from build123d import *

# Parameters (mm, degrees)
BOSS_EXTRUDE1_DEPTH   = 7.2
SKETCH1_3_R           = 3.75
SKETCH1_3_R_2         = 1.6
BOSS_EXTRUDE2_DEPTH   = 2
BOSS_EXTRUDE2_2_DEPTH = 2
BOSS_EXTRUDE3_DEPTH   = 2
BOSS_EXTRUDE4_DEPTH   = 7.5
SKETCH3_R             = 3.75
CUT_EXTRUDE6_DEPTH    = 12
BOSS_EXTRUDE5_DEPTH   = 7.5
SKETCH5_R             = 3.75
CUT_EXTRUDE7_DEPTH    = 7.5
SKETCH6_W             = 29.5
SKETCH6_H             = 8.4
BOSS_EXTRUDE6_DEPTH   = 4.3
SKETCH7_W             = 7.5
SKETCH7_H             = 7.2
SKETCH7_W_2           = 16.3
BOSS_EXTRUDE7_DEPTH   = 2
SKETCH8_W             = 10.1
SKETCH8_H             = 2.3
CUT_EXTRUDE8_DEPTH    = 12
SKETCH9_W             = 10.1
SKETCH9_H             = 1.2
BOSS_EXTRUDE8_DEPTH   = 6.4
SKETCH11_W            = 9.1347476
SKETCH11_H            = 5.173710516
BOSS_EXTRUDE11_DEPTH  = 5.5
SKETCH12_R            = 3.106234899
CUT_EXTRUDE10_DEPTH   = 1.5
CUT_EXTRUDE10_DRAFT   = -25
SKETCH13_R            = 3.196774454
CUT_EXTRUDE11_DEPTH   = 1.5
CUT_EXTRUDE11_DRAFT   = -29
SKETCH14_W            = 8.1347476
SKETCH14_H            = 4.5
CUT_EXTRUDE12_DEPTH   = 4.5
SCALE1_SCALE          = 0.2


# Read off the part's stored shape, not the designer's step: Dome1, Dome2
with BuildPart() as part:
    # Sketch1 → Boss-Extrude1 (new body)
    with BuildSketch(Plane(origin=(0, 0, 0), x_dir=(1, 0, 0), z_dir=(0, 1, 0))):
        Polygon((14.75, 0), (-14.75, 0), (-14.75, -3.75), (-14.75, -6.5), (14.75, -6.5), (14.75, -3.75), align=None)
        Polygon((-14.75, 3.75), (-14.75, 0), (14.75, 0), (14.75, 3.75), (14.75, 6.5), (-14.75, 6.5), align=None)
    extrude(amount=BOSS_EXTRUDE1_DEPTH)



with BuildPart() as body_2:
    # Sketch1<3> → Boss-Extrude2 (new body)
    with BuildSketch(Plane(origin=(0, 0, 0), x_dir=(1, 0, 0), z_dir=(0, 1, 0))):
        with Locations(Location((-18.5, 0, 0), (0, 0, 270))):
            Circle(SKETCH1_3_R)
        with Locations(Location((-18.5, 0, 0), (0, 0, 270))):
            Circle(SKETCH1_3_R_2, mode=Mode.SUBTRACT)
    extrude(amount=BOSS_EXTRUDE2_DEPTH)


with BuildPart() as body_3:
    # Sketch1<3> → Boss-Extrude2 2 (new body)
    with BuildSketch(Plane(origin=(0, 0, 0), x_dir=(1, 0, 0), z_dir=(0, 1, 0))):
        with Locations(Location((18.5, 0, 0), (0, 0, 270))):
            Circle(SKETCH1_3_R)
        with Locations(Location((18.5, 0, 0), (0, 0, 270))):
            Circle(SKETCH1_3_R_2, mode=Mode.SUBTRACT)
    extrude(amount=BOSS_EXTRUDE2_2_DEPTH)


with BuildPart() as part_1:
    add(part.part)

    add(body_2.part)  # Boss-Extrude3 merges body 2

    add(body_3.part)  # Boss-Extrude3 merges body 3
    # Sketch1<4> → Boss-Extrude3 (add)
    with BuildSketch(Plane(origin=(0, 0, 0), x_dir=(1, 0, 0), z_dir=(0, 1, 0))):
        with BuildLine():
            Line((-14.75, -3.75), (-14.75, 0))
            ThreePointArc((-14.75, 0), (-15.848349571, -2.651650429), (-18.5, -3.75))
            Line((-18.5, -3.75), (-14.75, -3.75))
        make_face()
        with BuildLine():
            Line((-14.75, 0), (-14.75, 3.75))
            Line((-14.75, 3.75), (-18.5, 3.75))
            ThreePointArc((-18.5, 3.75), (-15.848349571, 2.651650429), (-14.75, 0))
        make_face()
        with BuildLine():
            Line((18.5, 3.75), (14.75, 3.75))
            Line((14.75, 3.75), (14.75, 0))
            ThreePointArc((14.75, 0), (15.848349571, 2.651650429), (18.5, 3.75))
        make_face()
        with BuildLine():
            ThreePointArc((18.5, -3.75), (15.848349571, -2.651650429), (14.75, 0))
            Line((14.75, 0), (14.75, -3.75))
            Line((14.75, -3.75), (18.5, -3.75))
        make_face()
    extrude(amount=BOSS_EXTRUDE3_DEPTH)

    # Sketch2 → Boss-Extrude4 (add)
    with BuildSketch(Plane.XY.offset(3.75)):
        Polygon((18.5, 2), (14.75, 2), (14.75, 5.75), align=None)
    extrude(amount=-BOSS_EXTRUDE4_DEPTH)

    # Sketch3 → Cut-Extrude6 (cut)
    with BuildSketch(Plane(origin=(0, 2, 0), x_dir=(1, 0, 0), z_dir=(0, 1, 0))):
        with Locations((18.5, 0)):
            Circle(SKETCH3_R)
    extrude(amount=CUT_EXTRUDE6_DEPTH, mode=Mode.SUBTRACT)

    # Sketch4 → Boss-Extrude5 (add)
    with BuildSketch(Plane.XY.offset(3.75)):
        Polygon((-14.75, 5.75), (-18.5, 2), (-14.75, 2), align=None)
    extrude(amount=-BOSS_EXTRUDE5_DEPTH)

    # Sketch5 → Cut-Extrude7 (cut)
    with BuildSketch(Plane(origin=(0, 2, 0), x_dir=(1, 0, 0), z_dir=(0, 1, 0))):
        with Locations((-18.5, 0)):
            Circle(SKETCH5_R)
    extrude(amount=CUT_EXTRUDE7_DEPTH, mode=Mode.SUBTRACT)

    # Sketch6 → Boss-Extrude6 (add)
    with BuildSketch(Plane(origin=(0, 7.2, 0), x_dir=(1, 0, 0), z_dir=(0, 1, 0))):
        Rectangle(SKETCH6_W, SKETCH6_H)
    extrude(amount=BOSS_EXTRUDE6_DEPTH)

    # Sketch7 → Boss-Extrude7 (add)
    with BuildSketch(Plane(origin=(0, 11.5, 0), x_dir=(1, 0, 0), z_dir=(0, 1, 0))):
        with Locations((-10.25, 0)):
            Rectangle(SKETCH7_W, SKETCH7_H)
        with Locations((5.8, 0)):
            Rectangle(SKETCH7_W_2, SKETCH7_H)
    extrude(amount=BOSS_EXTRUDE7_DEPTH)

    # Sketch8 → Cut-Extrude8 (cut)
    with BuildSketch(Plane(origin=(0, 7.2, 0), x_dir=(1, 0, 0), z_dir=(0, 1, 0))):
        with Locations((0.003829246, -5.35)):
            Rectangle(SKETCH8_W, SKETCH8_H)
    extrude(amount=-CUT_EXTRUDE8_DEPTH, mode=Mode.SUBTRACT)

    # Sketch9 → Boss-Extrude8 (add)
    with BuildSketch(Plane.XY.offset(4.2)):
        with Locations((0.003829246, 3.9)):
            Rectangle(SKETCH9_W, SKETCH9_H)
    extrude(amount=BOSS_EXTRUDE8_DEPTH)

    # Sketch11 → Boss-Extrude11 (add)
    with BuildSketch(Plane(origin=(0, 4.5, 0), x_dir=(1, 0, 0), z_dir=(0, 1, 0))):
        with Locations((0.014014126, -7.894862881)):
            Rectangle(SKETCH11_W, SKETCH11_H)
    extrude(amount=BOSS_EXTRUDE11_DEPTH)


with BuildPart() as cut_extrude10_tool:
    # Sketch12 → Cut-Extrude10 (with draft: the straight prism first)
    with BuildSketch(Plane(origin=(0, 13.5, 0), x_dir=(1, 0, 0), z_dir=(0, 1, 0))):
        with Locations((-10.25, 0)):
            Circle(SKETCH12_R)
    extrude(amount=-CUT_EXTRUDE10_DEPTH)
    # Cut-Extrude10: the draft: its side faces are tilted about the plane it starts from
    cut_extrude10_sides = [cut_extrude10_tool.faces().sort_by_distance(p)[0] for p in [
        (-13.356234899, 12.75, 0),
    ]]
    draft(cut_extrude10_sides, Plane(origin=(0, 13.5, 0), x_dir=(1, 0, 0), z_dir=(0, 1, 0)), CUT_EXTRUDE10_DRAFT)


with BuildPart() as part_2:
    add(part_1.part)

    # Cut-Extrude10: cut by cut_extrude10_tool
    add(cut_extrude10_tool.part, mode=Mode.SUBTRACT)


with BuildPart() as cut_extrude11_tool:
    # Sketch13 → Cut-Extrude11 (with draft: the straight prism first)
    with BuildSketch(Plane(origin=(0, 13.5, 0), x_dir=(1, 0, 0), z_dir=(0, 1, 0))):
        with Locations((9.516994158, 0)):
            Circle(SKETCH13_R)
    extrude(amount=-CUT_EXTRUDE11_DEPTH)
    # Cut-Extrude11: the draft: its side faces are tilted about the plane it starts from
    cut_extrude11_sides = [cut_extrude11_tool.faces().sort_by_distance(p)[0] for p in [
        (6.320219704, 12.75, 0),
    ]]
    draft(cut_extrude11_sides, Plane(origin=(0, 13.5, 0), x_dir=(1, 0, 0), z_dir=(0, 1, 0)), CUT_EXTRUDE11_DRAFT)


with BuildPart() as part_3:
    add(part_2.part)

    # Cut-Extrude11: cut by cut_extrude11_tool
    add(cut_extrude11_tool.part, mode=Mode.SUBTRACT)

    # Dome1 outline → Dome1 (revolve)
    with BuildSketch(Plane(origin=(-10.25, 0, 0), x_dir=(1, 0, 0), z_dir=(0, 0, 1))):
        with BuildLine():
            Line((0, 12), (2.406773413, 11.999999998))
            ThreePointArc((2.406773413, 11.999999998), (1.417970228, 13.094302608), (0, 13.5))
            Line((0, 13.5), (0, 12))
        make_face()
    revolve(axis=Axis((-10.25, 0, 0), (0, 1, 0)))

    # Dome2 outline → Dome2 (revolve)
    with BuildSketch(Plane(origin=(9.516994158, 0, 0), x_dir=(1, 0, 0), z_dir=(0, 0, 1))):
        with BuildLine():
            Line((0, 12), (2.365310878, 11.999999998))
            ThreePointArc((2.365310878, 11.999999998), (1.400419183, 13.093385967), (0, 13.5))
            Line((0, 13.5), (0, 12))
        make_face()
    revolve(axis=Axis((9.516994158, 0, 0), (0, 1, 0)))

    # Sketch14 → Cut-Extrude12 (cut)
    with BuildSketch(Plane.XY.offset(10.481718139)):
        with Locations((0.014014126, 7.25)):
            Rectangle(SKETCH14_W, SKETCH14_H)
    extrude(amount=-CUT_EXTRUDE12_DEPTH, mode=Mode.SUBTRACT)


with BuildPart() as part_4:
    # Scale1: scaled about (0, 0, 0)
    add(part_3.part.scale(SCALE1_SCALE))


solid = part_4.part
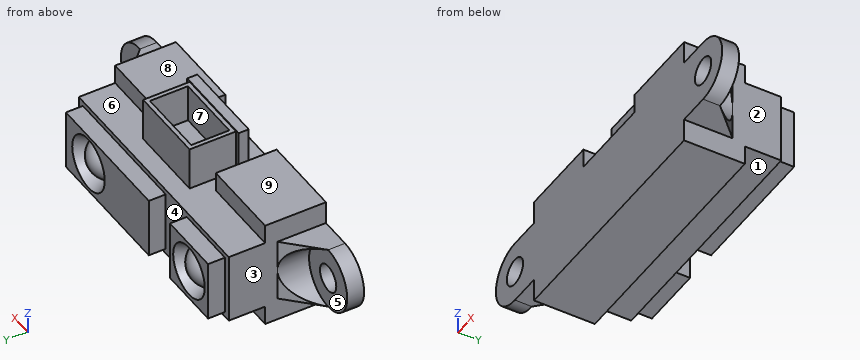
Part model, mm, in its own coordinate system. Face numbers are marked on the shaded views. A direction names the side the tool comes from. Round coordinates to 2 decimals unless told otherwise and drop trailing zeros. Write each loop counter-clockwise with the first axis right and the second up, starting at its lowest first coordinate (ties: lowest second). Pieces come first, ordered by that corner, then holes. Notation, with made-up numbers: (15, 36) - (74, 36) arc R37 ccw to (74, 74) - close; hole circle Ø5 at (18.5, 11). An arc over 180 degrees is marked (long way). Use CSV: the item, a comma, the result in double quotes.
Item 1: Pull direction X, two halves, no side cores. Call the marked faces 1, 2, 3 and 4: pulls with the +X half, pulls with the -X half, needs draft (parallel to the pull), parting line crosses it, or undercut.
Results list:
face 1,"needs draft"
face 2,"pulls with the +X half"
face 3,"pulls with the -X half"
face 4,"undercut"
Item 2: Slice it at B-B, the plane x = -2.05. Write the cut outline in (y, z).
Results list:
outline,"(0, -1.3) - (1.44, -1.3) - (1.44, -0.84) - (2.3, -0.84) - (2.3, -0.72) - (2.7, -0.72) - (2.7, -0.62) - (2.4, -0.48) arc R0.54 ccw to (2.4, 0.48) - (2.7, 0.62) - (2.7, 0.72) - (2.3, 0.72) - (2.3, 0.84) - (1.44, 0.84) - (1.44, 1.3) - (0, 1.3) - close"
Item 3: Slice it at A-A, the plane y = 1.55. Write the cut outline in (x, z), then the cut area to 3 significant figures.
Results list:
outline,"(-2.95, -0.84) - (2.95, -0.84) - (2.95, 0.84) - (-2.95, 0.84) - close; (-0.91, 1.06) - (0.92, 1.06) - (0.92, 2.1) - (0.82, 2.1) - (0.82, 1.2) - (-0.81, 1.2) - (-0.81, 2.1) - (-0.91, 2.1) - close"
area,"10.3 mm²"
Item 4: Wall check: L1, parallel to X at y = 0.2, z = 0; L2, parallel to Z at x = -3.7, y = 0.25; L3, parallel to Z at x = -1.5, y = 0.6. Give the ranges that are in metal, low to high.
Results list:
L1,"x = -4.45 to -4.02, -3.38 to 3.38, 4.02 to 4.45"
L2,"z = -0.75 to -0.32, 0.32 to 0.75"
L3,"z = -1.3 to 1.3"
Item 5: Tool access for the marked faces 5, 6, 7, 8 and 9: list every direction of +Z, -Z, +X, -X, +Y, -Y with a clear straight run to the whole face (end or side of a thin tool).
Results list:
face 5,"-X, +Y"
face 6,"+Y"
face 7,"+Z"
face 8,"+Z, +X, +Y, -Y"
face 9,"+Z, -X, +Y, -Y"
Item 6: Flat gauge pins, fed straight in: P1, Ø0.7, axis at x = -1.5, y = 1.5, coming from the +Z side; P2, Ø1.5, axis at x = -1.5, y = 0.5, coming from the +Z side; P3, Ø0.5, axis at x = -2, z = 1, coming from the +Y side; P4, Ø0.5, axis at y = 1.5, z = 2, coming from the +X side. Where does each tip first touch, or does it go through?
Results list:
P1,"stops at z = 1.3"
P2,"stops at z = 2.12"
P3,"stops at y = 2.3"
P4,"stops at x = 0.92"
Item 7: Slice it at D-D, the plane z = -1.1. Write the cut outline in (x, y), then the cut area to 3 significant figures.
Results list:
outline,"(-2.95, 0) - (2.95, 0) - (2.95, 1.44) - (-2.95, 1.44) - close"
area,"8.50 mm²"
Item 8: Slice it at C-C, the plane y = 0.25. Write the cut outline in (x, z), then the cut area to 3 significant figures.
Results list:
outline,"(-3.7, -0.75) - (-2.95, -0.75) - (-2.95, -1.3) - (2.95, -1.3) - (2.95, -0.75) - (3.7, -0.75) arc R0.75 ccw to (3.7, 0.75) - (2.95, 0.75) - (2.95, 1.3) - (1.01, 1.3) - (1.01, 0.84) - (-1.01, 0.84) - (-1.01, 1.3) - (-2.95, 1.3) - (-2.95, 0.75) - (-3.7, 0.75) arc R0.75 ccw to start; hole circle Ø0.64 at (-3.7, 0); hole circle Ø0.64 at (3.7, 0)"
area,"17.8 mm²"
